Design review of the part built by this model. Coordinates are the model's own, in mm. A direction names the side the tool comes from. Coordinates: 2 decimals unless noted, no trailing zeros. Order: outer loops, then holes, each group sorted by start corner. A loop starts at its lowest first (then second) coordinate and runs counter-clockwise, first axis right, second up. Notation, with made-up numbers: (62.5, 36.5) -> (94.5, 36.5) arc R35 ccw to (94.5, 72.5) -> close; hole circle Ø5 at (56.25, 30.5). An arc over 180 degrees is marked (long way). Use a Markdown table: item, result. Add a question column.
Q1. Machinability: for faces 5 (the face through (25.12, 3.54, 4.44)), 6 (the face through (42.715, 9.225, -1.521)), which of the approach directions +Z, -Z, +X, -X, +Y, -Y give a long, thin tool a straight path to every point of the face, cutting with its end or side? Answer none if there is none.
Q2. Insertion check: pin 1 (3 mm diameter, centred on x = 12, y = 4.5, fed in from +Z); pin 2 (1.4 mm diameter, centred on x = 42, y = 9, fed in from +Z). Each pin has a flat end and moves straight along its axis. Give the tip position at first contact, or say it passes through.
Q3. Add section B-B (x = 36.5). State the section outline as (y, z) points.
Q4. The part is to be moulded in two halves that separate along X. For faces 1 (the face through (0, 9, 3)), 2 (the face through (23, 0, 3)), 3 (the face through (24.69, 14.49, 4.44)), 4 (the face through (11, 4.1, -1.5)), say which applies: pulls with the +X half, pulls with the -X half, needs draft (parallel to the pull), parting line crosses it, or undercut.
Q5. Add section D-D (x = 44). State the section outline as (y, z) points.
Q6. Wall thickness on probe 1 along X at (y, z) = (8.75, 1.5); probe 2 along Y at (x, z) = (36.5, -1.3); probe 3 along Y at (x, z) = (6, -0.75): over which ranges is each line inside the solid? List them lowest first.
Q7. Add section C-C (y = 12.75). State the section outline as (x, z) points.
Q8. Add section A-A (z = 6.75). State the section outline as (x, y) points.
from build123d import *

# Parameters (mm, degrees)
BOSS_EXTRU_1_DEPTH = 9
BOSS_EXTRU_2_START = -3
ESQUISSE2_W        = 47
ESQUISSE2_H        = 18
ESQUISSE2_R        = 0.75
ESQUISSE2_R_2      = 5.5
BOSS_EXTRU_2_DEPTH = 3


with BuildPart() as part:
    # Esquisse1 → Boss.-Extru.1 (new body)
    with BuildSketch(Plane.XY):
        with BuildLine():
            Line((0, 18), (0, 9))
            Line((0, 9), (2, 9))
            ThreePointArc((2, 9), (3.903805922, 13.596194078), (8.5, 15.5))
            ThreePointArc((8.5, 15.5), (8.90545886, 15.48734176), (9.309338521, 15.449416342))
            Line((9.309338521, 15.449416342), (40.5, 13.5))
            ThreePointArc((40.5, 13.5), (43.681980515, 12.181980515), (45, 9))
            Line((45, 9), (47, 9))
            Line((47, 9), (47, 18))
            Line((47, 18), (0, 18))
        make_face()
        with BuildLine():
            Line((0, 9), (0, 0))
            Line((0, 0), (47, 0))
            Line((47, 0), (47, 9))
            Line((47, 9), (45, 9))
            ThreePointArc((45, 9), (43.681980515, 5.818019485), (40.5, 4.5))
            Line((40.5, 4.5), (9.309338521, 2.550583658))
            ThreePointArc((9.309338521, 2.550583658), (8.90545886, 2.51265824), (8.5, 2.5))
            ThreePointArc((8.5, 2.5), (3.903805922, 4.403805922), (2, 9))
            Line((2, 9), (0, 9))
        make_face()
    extrude(amount=BOSS_EXTRU_1_DEPTH)

    # Esquisse2 → Boss.-Extru.2 (add)
    with BuildSketch(Plane.XY.offset(BOSS_EXTRU_2_START)):
        with Locations((23.5, 9)):
            Rectangle(ESQUISSE2_W, ESQUISSE2_H)
        with BuildLine():
            Line((8.5, 2.5), (9.309338521, 2.550583658))
            ThreePointArc((9.309338521, 2.550583658), (8.90545886, 2.51265824), (8.5, 2.5))
        make_face(mode=Mode.SUBTRACT)
        with Locations((36.5, 9)):
            Circle(ESQUISSE2_R, mode=Mode.SUBTRACT)
        with Locations((31, 9)):
            Circle(ESQUISSE2_R, mode=Mode.SUBTRACT)
        with Locations((8.5, 9)):
            Circle(ESQUISSE2_R_2, mode=Mode.SUBTRACT)
        with BuildLine():
            Line((9.309338521, 15.449416342), (8.5, 15.5))
            ThreePointArc((8.5, 15.5), (8.90545886, 15.48734176), (9.309338521, 15.449416342))
        make_face(mode=Mode.SUBTRACT)
        with Locations((42, 9)):
            Circle(ESQUISSE2_R, mode=Mode.SUBTRACT)
    extrude(amount=BOSS_EXTRU_2_DEPTH)


solid = part.part
Established:
| question | item | result |
|---|---|---|
| 1 | face 5 | +Z |
| 1 | face 6 | +Z, -Z |
| 2 | pin 1 | z = 0 |
| 2 | pin 2 | through |
| 3 | outline | (0, -3) -> (8.25, -3) -> (8.25, 0) -> (4.25, 0) -> (4.25, 9) -> (0, 9) -> close; (9.75, -3) -> (18, -3) -> (18, 9) -> (13.75, 9) -> (13.75, 0) -> (9.75, 0) -> close |
| 4 | face 1 | pulls with the -X half |
| 4 | face 2 | needs draft |
| 4 | face 3 | undercut |
| 4 | face 4 | undercut |
| 5 | outline | (0, -3) -> (18, -3) -> (18, 9) -> (11.83, 9) -> (11.83, 0) -> (6.17, 0) -> (6.17, 9) -> (0, 9) -> close |
| 6 | probe 1 | 0 to 2, 44.99 to 47 |
| 6 | probe 2 | 0 to 8.25, 9.75 to 18 |
| 6 | probe 3 | 0 to 4.1, 13.9 to 18 |
| 7 | outline | (0, -3) -> (4.48, -3) -> (4.48, 0) -> (3.19, 0) -> (3.19, 9) -> (0, 9) -> close; (12.52, -3) -> (47, -3) -> (47, 9) -> (42.99, 9) -> (42.99, 0) -> (12.52, 0) -> close |
| 8 | outline | (0, 0) -> (47, 0) -> (47, 18) -> (0, 18) -> close; hole (9.31, 2.55) -> (40.5, 4.5) arc R4.5 ccw to (40.5, 13.5) -> (9.31, 15.45) arc R6.5 ccw (long way) to start |
